```python
from build123d import *

# Parameters (mm, degrees)
F0_W           = 13.97
F0_H           = 13.97
F1_DEPTH       = 25.4
F2_R           = 5.08
F3_DEPTH       = 2.54
F5_R           = 1.27
F6_W           = 15.875
F6_H           = 15.875
F7_DEPTH       = 2.54
F8_R           = 1.27
F9_R           = 0.762
F4_R           = 1.7145
F10_DEPTH      = 25.401
F10_DEPTH_BACK = 2.541
F11_W          = 17.78
F11_H          = 17.78
F11_W_2        = 11.43
F11_H_2        = 11.43
F12_DEPTH      = 12.7


with BuildPart() as f1:
    # F0 (on Top) → F1 (new body)
    with BuildSketch(Plane.XY):
        Rectangle(F0_W, F0_H)
    extrude(amount=F1_DEPTH)

    # F2 (on face) → F3 (cut)
    with BuildSketch(Plane.XY.offset(25.4)):
        Circle(F2_R)
    extrude(amount=-F3_DEPTH, mode=Mode.SUBTRACT)

    # F5
    f5_edges = [f1.edges().sort_by_distance(p)[0] for p in [
        (-6.985, 6.985, 12.7),
        (-6.985, -6.985, 12.7),
        (6.985, 6.985, 12.7),
        (6.985, -6.985, 12.7),
    ]]
    fillet(f5_edges, radius=F5_R)

    # F6 (on face) → F7 (join)
    with BuildSketch(Plane(origin=(0, 0, 0), x_dir=(1, 0, 0), z_dir=(0, 0, -1))):
        Rectangle(F6_W, F6_H)
    extrude(amount=F7_DEPTH)

    # F8
    f8_edges = [f1.edges().sort_by_distance(p)[0] for p in [
        (7.9375, -7.9375, -1.27),
        (-7.9375, -7.9375, -1.27),
        (-7.9375, 7.9375, -1.27),
        (7.9375, 7.9375, -1.27),
    ]]
    fillet(f8_edges, radius=F8_R)

    # F9
    f9_edges = [f1.edges().sort_by_distance(p)[0] for p in [
        (0, -7.9375, -2.54),
    ]]
    fillet(f9_edges, radius=F9_R)

    # F4 (on face) → F10 (cut, two sides)
    with BuildSketch(Plane(origin=(0, 0, 0), x_dir=(1, 0, 0), z_dir=(0, 0, -1))) as f10_sk:
        Circle(F4_R)
    extrude(amount=-F10_DEPTH, mode=Mode.SUBTRACT)
    extrude(f10_sk.sketch, amount=F10_DEPTH_BACK, mode=Mode.SUBTRACT)

    # F11 (on face) → F12 (cut)
    with BuildSketch(Plane.XY.offset(25.4)):
        Rectangle(F11_W, F11_H)
        Rectangle(F11_W_2, F11_H_2, mode=Mode.SUBTRACT)
    extrude(amount=-F12_DEPTH, mode=Mode.SUBTRACT)


solid = f1.part
```
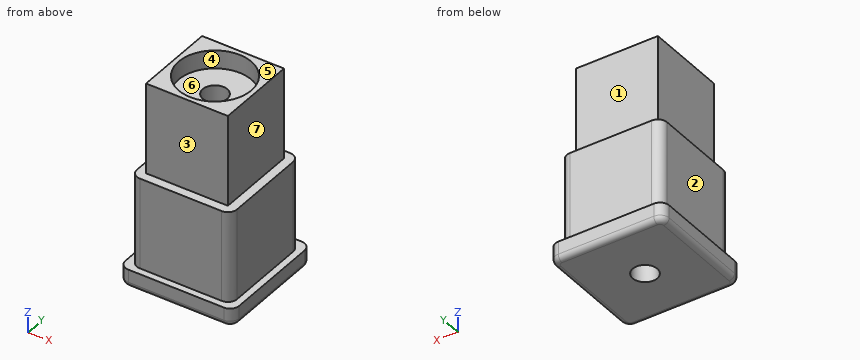
Work out the finished part from the listing and answer in its coordinate system (mm). Face numbers are marked on the shaded views. A direction names the side the tool comes from. Coordinates: 2 decimals unless noted, no trailing zeros. Loops run counter-clockwise (first coordinate to the right, second up) from the corner with the lowest first, then second, coordinate; pieces in that order, holes last. Notation, with made-up numbers: (19, 44.5) - (60, 44.5) arc R9 ccw to (60, 49.5) - close; hole circle Ø7 at (48, 84.25). An arc over 180 degrees is marked (long way). Use a Markdown table: item, result.
Item 1: The mould has two halves that part along X. Classify the marked faces 4, 5, 6 and 7: +X half, -X half, draft (parallel to the pull), parting line (faces both ways), or undercut.
Evaluation:
| item | result |
|---|---|
| face 4 | undercut |
| face 5 | draft |
| face 6 | undercut |
| face 7 | +X half |
Item 2: Consider probe 1 along Y at (x, z) = (0, 23.7) (3 decimals); probe 2 along X at (y, z) = (0, 15.5) (1 decimal); probe 3 along Y at (x, z) = (0, -1.35). Determine where each line is inside the solid, lowest interval first. Write a range as from..to.
Evaluation:
| item | result |
|---|---|
| probe 1 | y = -5.715..-5.08, 5.08..5.715 |
| probe 2 | x = -5.7..-1.7, 1.7..5.7 |
| probe 3 | y = -7.94..-1.71, 1.71..7.94 |
Item 3: Find section C-C, the plane z = 1.75. Determine the outline of the cut face in (x, y) (1 decimal).
Evaluation:
| item | result |
|---|---|
| outline | (-7, -5.7) arc R1.3 ccw to (-5.7, -7) - (5.7, -7) arc R1.3 ccw to (7, -5.7) - (7, 5.7) arc R1.3 ccw to (5.7, 7) - (-5.7, 7) arc R1.3 ccw to (-7, 5.7) - close; hole circle Ø3.4 at (0, 0) |
Item 4: Find section D-D, the plane y = 4.5. Determine the outline of the cut face in (x, z) (1 decimal), and give its area (3 significant figures).
Evaluation:
| item | result |
|---|---|
| outline | (-7.9, -1.8) arc R0.8 ccw to (-7.2, -2.5) - (7.2, -2.5) arc R0.8 ccw to (7.9, -1.8) - (7.9, 0) - (7, 0) - (7, 12.7) - (5.7, 12.7) - (5.7, 25.4) - (2.4, 25.4) - (2.4, 22.9) - (-2.4, 22.9) - (-2.4, 25.4) - (-5.7, 25.4) - (-5.7, 12.7) - (-7, 12.7) - (-7, 0) - (-7.9, 0) - close |
| area | 351 mm2 |
Item 5: Find section A-A, the plane x = 0. Determine the outline of the cut face in (y, z) (1 decimal), and give its area (3 significant figures).
Evaluation:
| item | result |
|---|---|
| outline | (-7.9, -1.8) arc R0.8 ccw to (-7.2, -2.5) - (-1.7, -2.5) - (-1.7, 22.9) - (-5.1, 22.9) - (-5.1, 25.4) - (-5.7, 25.4) - (-5.7, 12.7) - (-7, 12.7) - (-7, 0) - (-7.9, 0) - close; (1.7, -2.5) - (7.2, -2.5) arc R0.8 ccw to (7.9, -1.8) - (7.9, 0) - (7, 0) - (7, 12.7) - (5.7, 12.7) - (5.7, 25.4) - (5.1, 25.4) - (5.1, 22.9) - (1.7, 22.9) - close |
| area | 250 mm2 |
Item 6: For the marked faces 1, 2 and 3, determine the directions among +Z, -Z, +X, -X, +Y, -Y from which every point of the face is accessible in a straight line to the end or side of a thin tool.
Evaluation:
| item | result |
|---|---|
| face 1 | +Z, +X, -X, +Y |
| face 2 | +Z, -X, +Y, -Y |
| face 3 | +Z, +X, -X, -Y |
Item 7: Given pin 1 Ø5.5 at (y, z) = (0, 8.5) entering from +X (3 decimals); pin 2 Ø1.5 at (x, z) = (-1, 1) entering from -Y (3 decimals); pin 3 Ø5.5 at (x, z) = (-2, 20.5) entering from -Y (3 decimals), each flat-ended and moving along its own axis, determine where each tip first touches the part or whether it passes through.
Evaluation:
| item | result |
|---|---|
| pin 1 | stops at x = 6.985 |
| pin 2 | stops at y = -6.985 |
| pin 3 | stops at y = -5.715 |
